Source: CAD feature listing. Evaluate the final solid. Frame: model axes, mm. A direction names the side the tool comes from. Round coordinates to 2 decimals unless told otherwise and drop trailing zeros. Loops run counter-clockwise (first coordinate to the right, second up) from the corner with the lowest first, then second, coordinate; pieces in that order, holes last.
(1) Section C-C, the plane y = 10. Return the cut outline in (x, z), plus the area to 3 significant figures.
(2) Section B-B, the plane x = 0. Return the cut outline in (y, z) (3 decimals).
(3) Material intervals for probe 1 along X at (y, z) = (2, 0); probe 2 along Y at (x, z) = (-9, 6.5); probe 3 along X at (y, z) = (9, 0.75), sorted ascending.
(4) First-contact query: pin 1 Ø1 at (x, z) = (-16, 2.5) entering from -Y. Flat tip, straight axial feed; report the tip coordinate or a pass-through.
(5) Mould query, pull axis X, two halves, no side actions, for faces 5 (the flat face through (0, 7, -8.55)), 6 (the cylindrical face through (-2.44, 7.16, -0.54)), 7 (the cylindrical face through (-7.863, 14.802, -0.089)). Classes: pulls with the +X half, pulls with the -X half, needs draft (parallel to the pull), parting line crosses it, or undercut.
(6) Set-up query: faces 1 (the flat face through (0, -1, -6.375)), 2 (the flat face through (0, 15, -6.375)), 3 (the flat face through (0, -1, 6.375)), 4 (the flat face through (0, 15, 6.375)). Return all of +Z, -Z, +X, -X, +Y, -Y with unobstructed straight access to the full face (end or side cutting, diameter ignored); none if empty.
```python
from build123d import *

# Parameters (mm, degrees)
SKETCH1_W           = 41.2
SKETCH1_H           = 17.1
BOSS_EXTRUDE1_DEPTH = 14.05
BOSS_EXTRUDE2_START = 2.5
SKETCH2_W           = 14.3
SKETCH2_H           = 12.75
BOSS_EXTRUDE2_DEPTH = 19.05
FILLET1_R           = 2.5
SKETCH3_R           = 2.5
CUT_EXTRUDE1_DEPTH  = 30.331979135


with BuildPart() as part:
    # Sketch1 → Boss-Extrude1 (new body)
    with BuildSketch(Plane(origin=(0, 0, 0), x_dir=(1, 0, 0), z_dir=(0, 1, 0))):
        Rectangle(SKETCH1_W, SKETCH1_H)
    extrude(amount=BOSS_EXTRUDE1_DEPTH)

    # Sketch2 → Boss-Extrude2 (add)
    with BuildSketch(Plane(origin=(0, 14.05, 0), x_dir=(1, 0, 0), z_dir=(0, 1, 0)).offset(BOSS_EXTRUDE2_START)):
        Rectangle(SKETCH2_W, SKETCH2_H)
    extrude(amount=-BOSS_EXTRUDE2_DEPTH)

    # Fillet1
    fillet1_edges = [part.edges().sort_by_distance(p)[0] for p in [
        (7.15, 0, 0),
        (-7.15, 0, 0),
        (-7.15, 14.05, 0),
        (7.15, 14.05, 0),
    ]]
    fillet(fillet1_edges, radius=FILLET1_R - 0.0001)  # a hair under: the kernel refuses the full size

    # Sketch3 → Cut-Extrude1 (cut, through all)
    with BuildSketch(Plane(origin=(0, 16.55, 0), x_dir=(1, 0, 0), z_dir=(0, 1, 0))):
        with Locations(Location((0, 0, 0), (0, 0, 270))):
            Circle(SKETCH3_R)
    extrude(amount=-CUT_EXTRUDE1_DEPTH, mode=Mode.SUBTRACT)


solid = part.part
```
Output values:
1. outline: (-20.6, -8.55) - (20.6, -8.55) - (20.6, 8.55) - (-20.6, 8.55) - close; hole circle Ø5 at (0, 0)
1. area: 685 mm2
2. outline: (-2.5, -6.375) - (0, -6.375) - (0, -8.55) - (14.05, -8.55) - (14.05, -6.375) - (16.55, -6.375) - (16.55, -2.5) - (-2.5, -2.5) - close; (-2.5, 2.5) - (16.55, 2.5) - (16.55, 6.375) - (14.05, 6.375) - (14.05, 8.55) - (0, 8.55) - (0, 6.375) - (-2.5, 6.375) - close
3. probe 1: x = -20.6 to -2.5, 2.5 to 20.6
3. probe 2: y = 0 to 14.05
3. probe 3: x = -20.6 to -2.38, 2.38 to 20.6
4. pin 1: stops at y = 0
5. face 5: needs draft
5. face 6: undercut
5. face 7: pulls with the -X half
6. face 1: -Z, +X, -X, -Y
6. face 2: -Z, +X, -X, +Y
6. face 3: +Z, +X, -X, -Y
6. face 4: +Z, +X, -X, +Y
